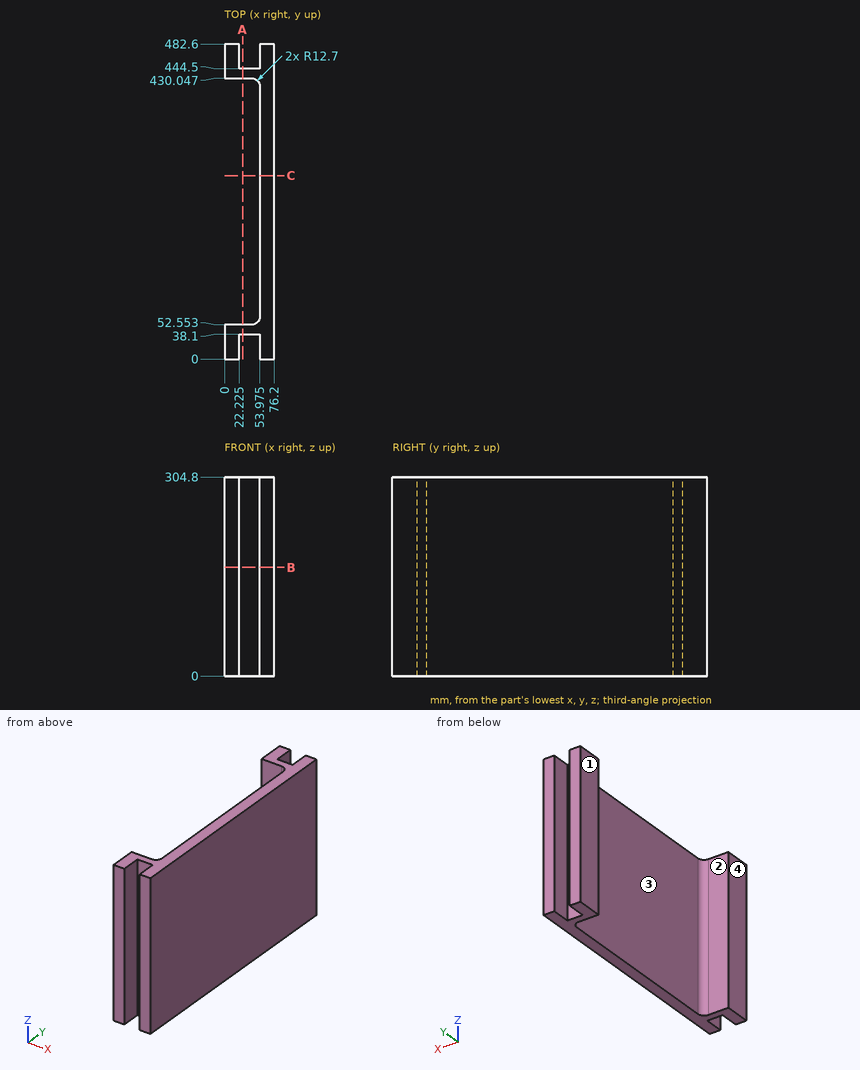
Could you check a few things on this drawing? It's one solid part, dimensions in mm from its lowest x, y, z. A direction names the side the tool comes from. Round coordinates to 2 decimals unless told otherwise and drop trailing zeros. Order: outer loops, then holes, each group sorted by start corner. A loop starts at its lowest first (then second) coordinate and runs counter-clockwise, first axis right, second up. Notation, with made-up numbers: M -38,51 L -11,51 A31 cw -11,82 Z; hole C 79,53.25 d1. An arc over 180 degrees is marked long. Return JSON: item names as keys, results as strings. Group by question number.
1. Please list where these lines run through material, in increasing order: probe 1 along Y at (x, z) = (8, 110.5); probe 2 along Y at (x, z) = (32.5, 107); probe 3 along X at (y, z) = (163, 72) (3 decimals).
2. If we section it at B-B on z = 166.5: List the corners of the cut face in (x, y) for me (3 decimals), then the cut area to 3 significant figures.
3. If we section it at C-C on y = 281: List the corners of the cut face in (x, z) for me (3 decimals).
4. If we section it at A-A on x = 27.5: List the corners of the cut face in (y, z) for me.
5. If we mould it in two halves opening along Y, with no side actions, what happens to the marked faces 1 and 2? For each: pulls with the +Y half, pulls with the -Y half, needs draft (parallel to the pull), parting line crosses it, or undercut.
6. I'm going to push flat-ended pins straight in: pin 1 Ø10 at (y, z) = (245.5, 101.5) entering from -X (3 decimals); pin 2 Ø2 at (x, z) = (34, 122.5) entering from -Y. Where does each tip first touch, or does it pass through?
7. On a 3-axis mill with a long thin cutter (end or side, diameter ignored), from which of +Z, -Z, +X, -X, +Y, -Y can I reach the whole of each face in a straight line? I mean the marked faces 3 and 4. Say none if no direction works.
Reply:
{
 "1": {"probe 1": "0 to 52.55, 430.05 to 482.6", "probe 2": "38.1 to 52.55, 430.05 to 444.5", "probe 3": "53.975 to 76.2"},
 "2": {"outline": "M 0,0 L 22.225,0 L 22.225,38.1 L 53.975,38.1 L 53.975,0 L 76.2,0 L 76.2,482.6 L 53.975,482.6 L 53.975,444.5 L 22.225,444.5 L 22.225,482.6 L 0,482.6 L 0,430.047 L 41.275,430.047 A12.7 cw 53.975,417.347 L 53.975,65.253 A12.7 cw 41.275,52.553 L 0,52.553 Z", "area": "14,000 mm^2"},
 "3": {"outline": "M 53.975,0 L 76.2,0 L 76.2,304.8 L 53.975,304.8 Z"},
 "4": {"outline": "M 38.1,0 L 52.55,0 L 52.55,304.8 L 38.1,304.8 Z; M 430.05,0 L 444.5,0 L 444.5,304.8 L 430.05,304.8 Z"},
 "5": {"face 1": "needs draft", "face 2": "undercut"},
 "6": {"pin 1": "x = 53.975", "pin 2": "y = 38.1"},
 "7": {"face 3": "+Z, -Z, -X", "face 4": "+Z, -Z, -X, +Y, -Y"}
}
